Read the model definition and answer for the solid it produces. Units are mm, in the model's axes. Coordinates: 2 decimals unless noted, no trailing zeros. Write each loop counter-clockwise with the first axis right and the second up, starting at its lowest first coordinate (ties: lowest second). Pieces come first, ordered by that corner, then holes.
Item 1: Straight lines are drawn through the part: probe 1 along Y at (x, z) = (-30, -21.5); probe 2 along Y at (x, z) = (-50, -12); probe 3 along X at (y, z) = (-49, -18.75). For each, find the intervals that lie inside material, in ascending order.
Item 2: Section A-A (y = 25) is taken. Give the vertices of the cut face in (x, z), then the cut area to 4 significant figures.
Item 3: Section C-C (x = -30) is taken. Give the vertices of the cut face in (y, z), then the cut area to 3 significant figures.
Item 4: Each of these flat-tipped pins is pushed along its axis until it touches: P1, Ø8, axis at x = -10.5, y = 96, coming from the +Z side; P2, Ø17.5, axis at x = 7.5, y = -96.5, coming from the +Z side. Where does it stop, or does it pass through?
Item 5: Section D-D (y = -97) is taken. Give the vertices of the cut face in (x, z), then the cut area to 3 significant figures.
Item 6: Section B-B (z = -7.75) is taken. State how many separate pieces and enclosed holes the cut face has, then the cut area to 3 significant figures.
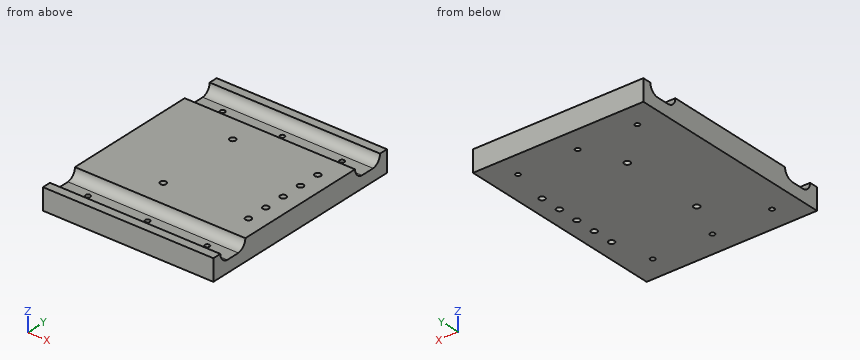
from build123d import *

# Parameters (mm, degrees)
F0_W     = 200
F0_H     = 10
F0_H_2   = 36
F0_R     = 2.75
F0_H_3   = 158
F0_R_2   = 3.5
F1_DEPTH = 25
F3_DEPTH = 200.001


with BuildPart() as f1:
    # F0 (on Top) → F1 (new body)
    with BuildSketch(Plane.XY):
        with Locations((-30, 120)):
            Rectangle(F0_W, F0_H)
        with Locations((-30, 97)):
            Rectangle(F0_W, F0_H_2)
        with Locations((-100, 97)):
            Circle(F0_R, mode=Mode.SUBTRACT)
        with Locations((-30, 97)):
            Circle(F0_R, mode=Mode.SUBTRACT)
        with Locations((40, 97)):
            Circle(F0_R, mode=Mode.SUBTRACT)
        with Locations((-30, 0)):
            Rectangle(F0_W, F0_H_3)
        with Locations((-50, -50)):
            Circle(F0_R_2, mode=Mode.SUBTRACT)
        with Locations((50, -50)):
            Circle(F0_R_2, mode=Mode.SUBTRACT)
        with Locations((50, -25)):
            Circle(F0_R_2, mode=Mode.SUBTRACT)
        with Locations((-50, 50)):
            Circle(F0_R_2, mode=Mode.SUBTRACT)
        with Locations((50, 0)):
            Circle(F0_R_2, mode=Mode.SUBTRACT)
        with Locations((50, 25)):
            Circle(F0_R_2, mode=Mode.SUBTRACT)
        with Locations((50, 50)):
            Circle(F0_R_2, mode=Mode.SUBTRACT)
        with Locations((-30, -97)):
            Rectangle(F0_W, F0_H_2)
        with Locations((-100, -97)):
            Circle(F0_R, mode=Mode.SUBTRACT)
        with Locations((-30, -97)):
            Circle(F0_R, mode=Mode.SUBTRACT)
        with Locations((40, -97)):
            Circle(F0_R, mode=Mode.SUBTRACT)
        with Locations((-30, -120)):
            Rectangle(F0_W, F0_H)
    extrude(amount=-F1_DEPTH)

    # F2 (on face) → F3 (cut, through all)
    with BuildSketch(Plane(origin=(-130, 0, 0), x_dir=(0, -1, 0), z_dir=(-1, 0, 0))):
        with BuildLine():
            Line((-79, 0), (-115, 0))
            ThreePointArc((-115, 0), (-112.126338, -7.433034), (-105, -11))
            Line((-105, -11), (-89, -11))
            ThreePointArc((-89, -11), (-81.873662, -7.433034), (-79, 0))
        make_face()
        with BuildLine():
            Line((115, 0), (79, 0))
            ThreePointArc((79, 0), (81.873662, -7.433034), (89, -11))
            Line((89, -11), (105, -11))
            ThreePointArc((105, -11), (112.126338, -7.433034), (115, 0))
        make_face()
    extrude(amount=-F3_DEPTH, mode=Mode.SUBTRACT)


solid = f1.part
Established:
1. probe 1: y = -125 to -99.75, -94.25 to 94.25, 99.75 to 125
1. probe 2: y = -125 to -53.5, -46.5 to 46.5, 53.5 to 125
1. probe 3: x = -130 to -53.35, -46.65 to 46.65, 53.35 to 70
2. outline: (-130, -25) - (46.5, -25) - (46.5, 0) - (-130, 0) - close; (53.5, -25) - (70, -25) - (70, 0) - (53.5, 0) - close
2. area: 4,825 mm2
3. outline: (-125, -25) - (-99.75, -25) - (-99.75, -11) - (-105, -11) arc R11.05 cw to (-115, 0) - (-125, 0) - close; (-94.25, -25) - (94.25, -25) - (94.25, -11) - (89, -11) arc R11.05 cw to (79, 0) - (-79, 0) arc R11.05 cw to (-89, -11) - (-94.25, -11) - close; (99.75, -25) - (125, -25) - (125, 0) - (115, 0) arc R11.05 cw to (105, -11) - (99.75, -11) - close
3. area: 5,410 mm2
4. P1: stops at z = -11
4. P2: stops at z = -10.81
5. outline: (-130, -25) - (-102.75, -25) - (-102.75, -11) - (-130, -11) - close; (-97.25, -25) - (-32.75, -25) - (-32.75, -11) - (-97.25, -11) - close; (-27.25, -25) - (37.25, -25) - (37.25, -11) - (-27.25, -11) - close; (42.75, -25) - (70, -25) - (70, -11) - (42.75, -11) - close
5. area: 2,570 mm2
6. separate pieces: 3
6. enclosed holes: 7
6. area: 37,900 mm2
